Input: part model. Units: mm. Frame: model coordinates. A direction names the side the tool comes from. Round coordinates to 2 decimals unless told otherwise and drop trailing zeros. Order: outer loops, then holes, each group sorted by start corner. A loop starts at its lowest first (then second) coordinate and runs counter-clockwise, first axis right, second up.
Item 1: Cut plane B-B on x = 25.5. Output: boundary loops of the cut face in (y, z), then the cut area to 3 significant figures.
Item 2: Reachability of faces 4 (the flat face through (34.9, 9.6, 1)), 5 (the flat face through (-28.38, 8, 0.99)) from +Z, -Z, +X, -X, +Y, -Y: full face, straight path, thin tool, end or side. Return the list, or none.
Item 3: Mould query, pull axis Y, two halves, no side actions, for faces 1 (the flat face through (-35.51, -10.87, 0.99)), 2 (the flat face through (-63.8, 9.7, 1)), 3 (the flat face through (-60.6, -12.9, 1)). Classes: released by +Y, released by -Y, zero draft, split by the parting line, or undercut.
Item 4: Cut plane D-D on y = 12.5. Output: boundary loops of the cut face in (x, z), then the cut area to 3 significant figures.
Item 5: Cut plane A-A on x = 14.35. Output: boundary loops of the cut face in (y, z).
Item 6: Cut plane C-C on z = 1.45. Give the number of separate pieces and of enclosed holes in the cut face, then the cut area to 3 significant figures.
Item 7: Line query: L1, parallel to Y at x = 14.35, z = 1.05; L2, parallel to Y at x = -1, z = 1.15; L3, parallel to Y at x = -3.5, z = 1. Output: solid intervals per line, ascending.
Item 8: First-contact query: pin 1 (0.6 mm diameter, centred on x = -60.5, z = 1.5, fed in from -Y). Flat tip, straight axial feed; report the tip coordinate or a pass-through.
```python
from build123d import *

# Parameters (mm, degrees)
SKETCH_1_W             = 32.7
SKETCH_1_H             = 29
SKETCH_1_R             = 1.5
EXTRUDE_1_DEPTH        = 2
CHAMFER_1_SIZE         = 3
EXTRUDE_2_DEPTH        = 2
CHAMFER_2_SIZE         = 9.5
EXTRUDE_3_DEPTH        = 2
SKETCH_6_R             = 1.6
CUT_EXTRUDE_2_DEPTH    = 72.529714105
CUT_EXTRUDE_4_DEPTH    = 10
FILLET_2_R             = 1
FILLET_2_OF_MIRROR_1_R = 1
SKETCH_8_W             = 55
SKETCH_8_H             = 35
CUT_EXTRUDE_5_DEPTH    = 72.529714105
EXTRUDE_4_DEPTH        = 2
CUT_EXTRUDE_6_DEPTH    = 72.529714105
FILLET_4_R             = 1


with BuildPart() as part:
    # 草图1 → 凸台-拉伸1 (new body)
    with BuildSketch(Plane.XY):
        Rectangle(SKETCH_1_W, SKETCH_1_H)
        with Locations((-14.35, -10)):
            Circle(SKETCH_1_R, mode=Mode.SUBTRACT)
        with Locations((-14.35, 10)):
            Circle(SKETCH_1_R, mode=Mode.SUBTRACT)
        with Locations((14.35, 10)):
            Circle(SKETCH_1_R, mode=Mode.SUBTRACT)
        with Locations((14.35, -10)):
            Circle(SKETCH_1_R, mode=Mode.SUBTRACT)
        with Locations((-14.35, 0)):
            Circle(SKETCH_1_R, mode=Mode.SUBTRACT)
        with Locations((14.35, 0)):
            Circle(SKETCH_1_R, mode=Mode.SUBTRACT)
    extrude(amount=EXTRUDE_1_DEPTH)

    # 倒角1
    chamfer_1_edges = [part.edges().sort_by_distance(p)[0] for p in [
        (16.35, -14.5, 1),
        (-16.35, -14.5, 1),
        (-16.35, 14.5, 1),
        (16.35, 14.5, 1),
    ]]
    chamfer(chamfer_1_edges, length=CHAMFER_1_SIZE)

    # 草图3 → 凸台-拉伸2 (add)
    with BuildSketch(Plane.XY.offset(2)):
        Polygon((-13.35, 14.5), (-68.5, 14.5), (-68.5, -14.5), (-13.35, -14.5), (-16.35, -11.5), (-16.35, 11.5), align=None)
        Polygon((68.5, 14.5), (13.35, 14.5), (16.35, 11.5), (16.35, -11.5), (13.35, -14.5), (68.5, -14.5), align=None)
    extrude(amount=-EXTRUDE_2_DEPTH)

    # 倒角2
    chamfer_2_edges = [part.edges().sort_by_distance(p)[0] for p in [
        (-68.5, -14.5, 1),
        (-68.5, 14.5, 1),
        (68.5, -14.5, 1),
        (68.5, 14.5, 1),
    ]]
    chamfer(chamfer_2_edges, length=CHAMFER_2_SIZE)

    # 草图4 → 凸台-拉伸3 (add)
    with BuildSketch(Plane(origin=(0, 0, 0), x_dir=(-1, 0, 0), z_dir=(0, 0, -1))):
        Polygon((-59, -14.5), (-53, -20.5), (53, -20.5), (59, -14.5), align=None)
    extrude(amount=-EXTRUDE_3_DEPTH)

    # 草图6 → 切除-拉伸2 (cut, through all)
    with BuildSketch(Plane(origin=(0, 0, 0), x_dir=(-1, 0, 0), z_dir=(0, 0, -1))):
        with Locations((-63.5, 0)):
            Circle(SKETCH_6_R)
    cut_extrude_2 = extrude(amount=-CUT_EXTRUDE_2_DEPTH, mode=Mode.SUBTRACT)

    # 草图7 → 切除-拉伸4 (cut)
    with BuildSketch(Plane(origin=(0, 0, 0), x_dir=(-1, 0, 0), z_dir=(0, 0, -1))):
        Polygon((-57, 11.5), (-65.5, 3), (-57.621320344, 3), (-49.121320344, 11.5), align=None)
        Polygon((-57.621320344, -3), (-65.5, -3), (-51, -17.5), (-43.121320344, -17.5), align=None)
        Polygon((-47.621320344, -3), (-53.378679656, -3), (-38.878679656, -17.5), (-33.121320344, -17.5), align=None)
        Polygon((-44.878679656, 11.5), (-53.378679656, 3), (-47.621320344, 3), (-39.121320344, 11.5), align=None)
        Polygon((-34.878679656, 11.5), (-43.378679656, 3), (-37.621320344, 3), (-29.121320344, 11.5), align=None)
        Polygon((-23.121320344, -17.5), (-37.621320344, -3), (-43.378679656, -3), (-28.878679656, -17.5), align=None)
        Polygon((-20, -8.5), (-25.5, -3), (-33.378679656, -3), (-20, -16.378679656), align=None)
        Polygon((-33.378679656, 3), (-25.5, 3), (-20, 8.5), (-20, 11.5), (-23, 11.5), (-24.878679656, 11.5), align=None)
    cut_extrude_4 = extrude(amount=-CUT_EXTRUDE_4_DEPTH, mode=Mode.SUBTRACT)

    # 圆角2
    fillet_2_edges = [part.edges().sort_by_distance(p)[0] for p in [
        (53.378679656, -3, 1),
        (47.621320344, -3, 1),
        (33.121320344, -17.5, 1),
        (38.878679656, -17.5, 1),
        (57.621320344, -3, 1),
        (43.121320344, -17.5, 1),
        (51, -17.5, 1),
        (65.5, -3, 1),
        (37.621320344, 3, 1),
        (43.378679656, 3, 1),
        (34.878679656, 11.5, 1),
        (29.121320344, 11.5, 1),
        (47.621320344, 3, 1),
        (53.378679656, 3, 1),
        (44.878679656, 11.5, 1),
        (39.121320344, 11.5, 1),
        (33.378679656, -3, 1),
        (25.5, -3, 1),
        (20, -8.5, 1),
        (20, -16.378679656, 1),
        (43.378679656, -3, 1),
        (37.621320344, -3, 1),
        (23.121320344, -17.5, 1),
        (28.878679656, -17.5, 1),
        (33.378679656, 3, 1),
        (24.878679656, 11.5, 1),
        (20, 11.5, 1),
        (20, 8.5, 1),
        (25.5, 3, 1),
        (57.621320344, 3, 1),
        (65.5, 3, 1),
        (57, 11.5, 1),
        (49.121320344, 11.5, 1),
    ]]
    fillet(fillet_2_edges, radius=FILLET_2_R)

    # 镜向1: 切除-拉伸2, 切除-拉伸4 across plane
    add(cut_extrude_2.mirror(Plane(origin=(0, 0, 0), x_dir=(0, 0, 1), z_dir=(1, 0, 0))), mode=Mode.SUBTRACT)
    add(cut_extrude_4.mirror(Plane(origin=(0, 0, 0), x_dir=(0, 0, 1), z_dir=(1, 0, 0))), mode=Mode.SUBTRACT)

    # 圆角2 of 镜向1
    fillet_2_of_mirror_1_edges = [part.edges().sort_by_distance(p)[0] for p in [
        (-53.378679656, -3, 1),
        (-47.621320344, -3, 1),
        (-33.121320344, -17.5, 1),
        (-38.878679656, -17.5, 1),
        (-57.621320344, -3, 1),
        (-43.121320344, -17.5, 1),
        (-51, -17.5, 1),
        (-65.5, -3, 1),
        (-37.621320344, 3, 1),
        (-43.378679656, 3, 1),
        (-34.878679656, 11.5, 1),
        (-29.121320344, 11.5, 1),
        (-47.621320344, 3, 1),
        (-53.378679656, 3, 1),
        (-44.878679656, 11.5, 1),
        (-39.121320344, 11.5, 1),
        (-33.378679656, -3, 1),
        (-25.5, -3, 1),
        (-20, -8.5, 1),
        (-20, -16.378679656, 1),
        (-43.378679656, -3, 1),
        (-37.621320344, -3, 1),
        (-23.121320344, -17.5, 1),
        (-28.878679656, -17.5, 1),
        (-33.378679656, 3, 1),
        (-24.878679656, 11.5, 1),
        (-20, 11.5, 1),
        (-20, 8.5, 1),
        (-25.5, 3, 1),
        (-57.621320344, 3, 1),
        (-65.5, 3, 1),
        (-57, 11.5, 1),
        (-49.121320344, 11.5, 1),
    ]]
    fillet(fillet_2_of_mirror_1_edges, radius=FILLET_2_OF_MIRROR_1_R)

    # 草图8 → 切除-拉伸5 (cut, through all)
    with BuildSketch(Plane.XY.offset(2)):
        with Locations((47.5, -3)):
            Rectangle(SKETCH_8_W, SKETCH_8_H)
    extrude(amount=-CUT_EXTRUDE_5_DEPTH, mode=Mode.SUBTRACT)

    # 草图9 → 凸台-拉伸4 (add)
    with BuildSketch(Plane.XY.offset(2)):
        Polygon((20, -20.5), (20, 14.5), (30, 14.5), (40, 4.5), (40, -10.5), (30, -20.5), align=None)
    extrude(amount=-EXTRUDE_4_DEPTH)

    # 草图10 → 切除-拉伸6 (cut, through all)
    with BuildSketch(Plane.XY.offset(2)):
        Polygon((9.082528349, 10.5), (-8.582528349, 10.5), (0.25, -0.592012346), align=None)
        Polygon((11, -14.092012346), (11, 8.092012346), (2.167471651, -3), align=None)
        Polygon((-1.667471651, -3), (-10.5, 8.092012346), (-10.5, -14.092012346), align=None)
        Polygon((0.25, -5.407987654), (-8.582528349, -16.5), (9.082528349, -16.5), align=None)
        Polygon((18, -16.5), (18, 10.5), (28.343145751, 10.5), (36, 2.843145751), (36, -8.843145751), (28.343145751, -16.5), align=None)
    extrude(amount=-CUT_EXTRUDE_6_DEPTH, mode=Mode.SUBTRACT)

    # 圆角4
    fillet_4_edges = [part.edges().sort_by_distance(p)[0] for p in [
        (2.167471651, -3, 1),
        (11, 8.092012346, 1),
        (11, -14.092012346, 1),
        (-10.5, 8.092012346, 1),
        (-1.667471651, -3, 1),
        (-10.5, -14.092012346, 1),
        (0.25, -5.407987654, 1),
        (9.082528349, -16.5, 1),
        (-8.582528349, -16.5, 1),
        (18, -16.5, 1),
        (18, 10.5, 1),
        (28.343145751, 10.5, 1),
        (36, 2.843145751, 1),
        (36, -8.843145751, 1),
        (28.343145751, -16.5, 1),
        (-8.582528349, 10.5, 1),
        (9.082528349, 10.5, 1),
        (0.25, -0.592012346, 1),
    ]]
    fillet(fillet_4_edges, radius=FILLET_4_R)


solid = part.part
```
From the geometry:
1. outline: (-20.5, 0) - (-16.5, 0) - (-16.5, 2) - (-20.5, 2) - close; (10.5, 0) - (14.5, 0) - (14.5, 2) - (10.5, 2) - close
1. area: 16.0 mm2
2. face 4: +Z, -Z, +X, +Y
2. face 5: +Z, -Z
3. face 1: undercut
3. face 2: released by +Y
3. face 3: released by -Y
4. outline: (-61, 0) - (32, 0) - (32, 2) - (-61, 2) - close
4. area: 186 mm2
5. outline: (-20.5, 0) - (-11.5, 0) - (-11.5, 2) - (-20.5, 2) - close; (-8.5, 0) - (-1.5, 0) - (-1.5, 2) - (-8.5, 2) - close; (1.5, 0) - (8.5, 0) - (8.5, 2) - (1.5, 2) - close; (11.5, 0) - (14.5, 0) - (14.5, 2) - (11.5, 2) - close
6. separate pieces: 1
6. enclosed holes: 20
6. area: 2,110 mm2
7. L1: y = -20.5 to -11.5, -8.5 to -1.5, 1.5 to 8.5, 11.5 to 14.5
7. L2: y = -20.5 to -16.5, -6.98 to 0.98, 10.5 to 14.5
7. L3: y = -20.5 to -16.5, -10.12 to -5.3, -0.7 to 4.12, 10.5 to 14.5
8. pin 1: stops at y = -13.3
